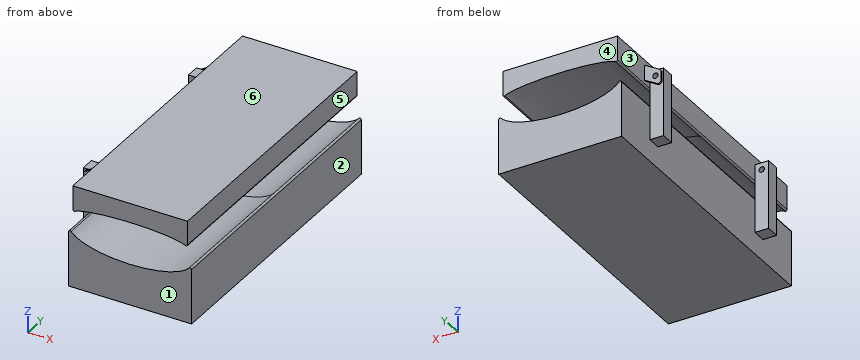
```python
from build123d import *

# Parameters (mm, degrees)
F1_DEPTH      = 1050
F1_DEPTH_BACK = 1050
F2_W          = 100
F2_H          = 256.5368058683
F2_H_2        = 243.4631941317
F3_DEPTH      = 100
F4_R          = 20
F5_DEPTH      = 1400
F7_DEPTH      = 1050
F7_DEPTH_BACK = 1050
F8_R          = 20
F9_DEPTH      = 15


with BuildPart() as f1:
    # F0 (on Front) → F1 (new body, two sides)
    with BuildSketch(Plane.XZ) as f1_sk:
        with BuildLine():
            Line((-450, 0), (0, 0))
            Line((0, 0), (450, 0))
            Line((450, 0), (450, 401.9604354327))
            ThreePointArc((450, 401.9604354327), (443.487330164, 411.3326565317), (432.4322943345, 408.4972413011))
            add(Edge.make_bspline(
                [(-432.4322943345, 408.4972413011), (4.257e-07, -92.1326371016), (432.4322943997, 408.4972413765)],
                knots=[3.4219354285, 3.4219354285, 3.4219354285, 6.0028425328, 6.0028425328, 6.0028425328], degree=2, weights=[1, 0.2766850577, 1]))
            ThreePointArc((-432.4322943345, 408.4972413011), (-443.487330164, 411.3326565317), (-450, 401.9604354327))
            Line((-450, 401.9604354327), (-450, 0))
        make_face()
    extrude(amount=F1_DEPTH)
    extrude(f1_sk.sketch, amount=-F1_DEPTH_BACK)

    # F2 (on face) → F3 (join)
    with BuildSketch(Plane(origin=(-450, 0, 0), x_dir=(0, -1, 0), z_dir=(-1, 0, 0))):
        with Locations((-650, 530.2288383669)):
            Rectangle(F2_W, F2_H)
        with Locations((-650, 280.2288383669)):
            Rectangle(F2_W, F2_H_2)
        with Locations((650, 280.2288383669)):
            Rectangle(F2_W, F2_H_2)
        with Locations((650, 530.2288383669)):
            Rectangle(F2_W, F2_H)
    extrude(amount=F3_DEPTH)

    # F4 (on face) → F5 (cut, through all)
    with BuildSketch(Plane.XZ.offset(700)):
        with Locations((-500, 608.4972413011)):
            Circle(F4_R)
    extrude(amount=-F5_DEPTH, mode=Mode.SUBTRACT)



with BuildPart() as f7:
    # F6 (on Front) → F7 (new body, two sides)
    with BuildSketch(Plane.XZ) as f7_sk:
        with BuildLine():
            Line((420, 750), (0, 750))
            Line((0, 750), (-420, 750))
            Line((-420, 750), (-420, 574.5617983004))
            ThreePointArc((-420, 574.5617983004), (-415.1679597445, 566.0007123834), (-405.3415615842, 565.7131288227))
            add(Edge.make_bspline(
                [(405.3415615842, 565.7131288227), (0, 779.1077760916), (-405.3415615842, 565.7131288227)],
                knots=[0.2649753519, 0.2649753519, 0.2649753519, 2.8766173017, 2.8766173017, 2.8766173017], degree=2, weights=[1, 0.2618854804, 1]))
            ThreePointArc((405.3415615842, 565.7131288227), (415.1679597445, 566.0007123834), (420, 574.5617983004))
            Line((420, 574.5617983004), (420, 750))
        make_face()
    extrude(amount=F7_DEPTH)
    extrude(f7_sk.sketch, amount=-F7_DEPTH_BACK)


with BuildPart() as f1_1:
    add(f1.part)

    add(f7.part)  # F9 merges F7
    # F8 (on face) → F9 (join)
    with BuildSketch(Plane.XZ.offset(700)):
        Polygon((-420, 600), (-420, 710), (-509.2053947965, 658.4972413011), (-450, 658.4972413011), (-450, 582.6794919243), align=None)
        with BuildLine():
            Line((-450, 658.4972413011), (-509.2053947965, 658.4972413011))
            Line((-509.2053947965, 658.4972413011), (-530, 646.4914703891))
            ThreePointArc((-530, 646.4914703891), (-537.3205080757, 639.1709623135), (-540, 629.1709623135))
            Line((-540, 629.1709623135), (-540, 565.3589838486))
            ThreePointArc((-540, 565.3589838486), (-530, 548.0384757729), (-510, 548.0384757729))
            Line((-510, 548.0384757729), (-450, 582.6794919243))
            Line((-450, 582.6794919243), (-450, 658.4972413011))
        make_face()
        with Locations((-500, 608.4972413011)):
            Circle(F8_R, mode=Mode.SUBTRACT)
    extrude(amount=F9_DEPTH)

    # F10: F1 across plane


with BuildPart() as f1_2:
    add(f1_1.part)
    add(f1_1.part.mirror(Plane.XZ))


solid = f1_2.part
```
Model file for the job. Use its own axes, mm. Face numbers are marked on the shaded views. A direction names the side the tool comes from. Give positions to 0.01 mm unless a question says otherwise; leave off trailing zeros. Order: outer loops, then holes, each group sorted by start corner. A loop starts at its lowest first (then second) coordinate and runs counter-clockwise, first axis right, second up.
1) Mould opens along Y. For the marked faces 1, 2, 3 and 4 say: +Y half, -Y half, draft (parallel to the pull), parting line (faces both ways), or undercut.
2) Wall check: probe 1 along Z at (x, y) = (10.5, -441); probe 2 along Z at (x, y) = (-500, -672); probe 3 along X at (y, z) = (907, 195). Give the ranges that are in metal, low to high.
3) Pin check, flat tip, straight feed: pin 1 (7.5 mm diameter, centred on y = 704, z = 595, fed in from -X). Stop position of the tip, or through.
4) Saw through at A-A, the plane y = 679. Count the separate pieces of the cut face and the enclosed holes in it, then the cut area to 3 significant figures.
5) Saw through at B-B, the plane z = 94. Write the cut outline in (x, y).
6) 3-axis set-ups, long thin cutter, end or side, ignore diameter. For the marked faces 5 and 6: which of +Z, -Z, +X, -X, +Y, -Y reach the whole face in a straight line?
Computed:
1. face 1: -Y half
1. face 2: draft
1. face 3: undercut
1. face 4: +Y half
2. probe 1: z = 0 to 300.04, 609.98 to 750
2. probe 2: z = 158.5 to 588.5, 628.5 to 658.5
2. probe 3: x = -450 to 450
3. pin 1: stops at x = -540
4. separate pieces: 2
4. enclosed holes: 1
4. area: 476,000 mm2
5. outline: (-450, -1050) - (450, -1050) - (450, 1050) - (-450, 1050) - close
6. face 5: +Z, +X, +Y, -Y
6. face 6: +Z, +X, -X, +Y, -Y
